Geometry: final body of the model. Coordinates: model frame, mm. A direction names the side the tool comes from. Give positions to 0.01 mm unless a question says otherwise; leave off trailing zeros. Loops run counter-clockwise (first coordinate to the right, second up) from the corner with the lowest first, then second, coordinate; pieces in that order, holes last. Notation, with made-up numbers: (-18.75, -5.75) -> (34.25, -5.75) arc R5 cw to (34.25, -1.75) -> close; hole circle Ø9 at (6.5, 17.25). An arc over 180 degrees is marked (long way). Answer in a Markdown table with one row per item. Add a question column.
1) Draft query along X for faces 1 (the flat face through (22.5, 51, -7)), 2 (the cylindrical face through (5.24, 58.166, -18.517)), 3 (the flat face through (1, 48, -18)). Return one class per face: +X half, -X half, draft (parallel to the pull), parting line (faces both ways), or undercut.
2) Section query A-A (z = -20.5). Return the cut outline in (x, y).
3) First-contact query: P1, Ø6.5, axis at x = 25.5, z = -20.5, coming from the +Y side; P2, Ø1, axis at y = 52.5, z = -14, coming from the +X side; P3, Ø1, axis at x = 9.5, z = -14.5, coming from the +Y side; P4, Ø2, axis at x = 20, y = 55.5, coming from the +Z side. Flat tips, straight axial feed; report the tip coordinate or a pass-through.
4) Line query: line 1 (X direction, y = 57.6, z = -20.5); line 2 (Y direction, x = 27, z = -18); line 3 (X direction, y = 52, z = -13.25). Output: solid intervals per line, ascending. Write a range as from..to.
5) Access query for faces 4 (the flat face through (3, 57, -21)), 5 (the flat face through (8.5, 58, -21)), 6 (the flat face through (5, 54, -27.5)), 7 (the flat face through (16, 52, -33.5)), 8 (the flat face through (5, 54, -16.5)). Directions: +Z, -Z, +X, -X, +Y, -Y. A direction counts if a zero-diameter tool reaches every point of the face in a straight line with its end or side. Return the directions, or none.
6) Section query D-D (x = 19.5). Return the cut outline in (y, z).
7) Section query C-C (x = 25.5). Return the cut outline in (y, z), plus the area to 3 significant figures.
8) Section query B-B (y = 54.25). Return the cut outline in (x, z).
```python
from build123d import *

# Parameters (mm, degrees)
BOX227_W          = 10
BOX227_H          = 10
BOX227_DEPTH      = 4
BOX217_W          = 13
BOX217_H          = 2
BOX217_DEPTH      = 1
BOX213_W          = 1
BOX213_H          = 2
BOX213_DEPTH      = 28
BOX210_W          = 2
BOX210_H          = 1
BOX210_DEPTH      = 28
BOX215_W          = 13
BOX215_H          = 2
BOX215_DEPTH      = 1
BOX212_W          = 12
BOX212_H          = 1
BOX212_DEPTH      = 2
BOX211_W          = 12
BOX211_H          = 1
BOX211_DEPTH      = 2
CYLINDER092_R     = 2
CYLINDER092_DEPTH = 5
CYLINDER093_R     = 4
CYLINDER093_DEPTH = 5
BOX073_W          = 30
BOX073_H          = 4
BOX073_DEPTH      = 30
FILLET057_R       = 6
CYLINDER088_R     = 2
CYLINDER088_DEPTH = 5
BOX221_W          = 6
BOX221_H          = 2.3
BOX221_DEPTH      = 14
FILLET055_R       = 2
BOX209_W          = 6
BOX209_H          = 7
BOX209_DEPTH      = 3
BOX222_W          = 6
BOX222_H          = 7
BOX222_DEPTH      = 3
FILLET059_R       = 1.5


with BuildPart() as cube215:
    # Box227 → Box227 (new body)
    with BuildSketch(Plane(origin=(28, 40, -16), x_dir=(1, 0, 0), z_dir=(0, 0, 1))):
        with Locations((5, 5)):
            Rectangle(BOX227_W, BOX227_H)
    extrude(amount=BOX227_DEPTH)


with BuildPart() as cube206:
    # Box217 → Box217 (new body)
    with BuildSketch(Plane(origin=(9.5, 51, -34.5), x_dir=(1, 0, 0), z_dir=(0, 0, 1))):
        with Locations((6.5, 1)):
            Rectangle(BOX217_W, BOX217_H)
    extrude(amount=BOX217_DEPTH)


with BuildPart() as cube202:
    # Box213 → Box213 (new body)
    with BuildSketch(Plane(origin=(8.5, 51, -34.5), x_dir=(1, 0, 0), z_dir=(0, 0, 1))):
        with Locations((0.5, 1)):
            Rectangle(BOX213_W, BOX213_H)
    extrude(amount=BOX213_DEPTH)


with BuildPart() as cube199:
    # Box210 → Box210 (new body)
    with BuildSketch(Plane(origin=(8.5, 50, -34.5), x_dir=(1, 0, 0), z_dir=(0, 0, 1))):
        with Locations((1, 0.5)):
            Rectangle(BOX210_W, BOX210_H)
    extrude(amount=BOX210_DEPTH)


with BuildPart() as cube204:
    # Box215 → Box215 (new body)
    with BuildSketch(Plane(origin=(9.5, 51, -7.5), x_dir=(1, 0, 0), z_dir=(0, 0, 1))):
        with Locations((6.5, 1)):
            Rectangle(BOX215_W, BOX215_H)
    extrude(amount=BOX215_DEPTH)


with BuildPart() as cube201:
    # Box212 → Box212 (new body)
    with BuildSketch(Plane(origin=(10.5, 50, -8.5), x_dir=(1, 0, 0), z_dir=(0, 0, 1))):
        with Locations((6, 0.5)):
            Rectangle(BOX212_W, BOX212_H)
    extrude(amount=BOX212_DEPTH)


with BuildPart() as fusion070:
    # Box211 → Box211 (new body)
    with BuildSketch(Plane(origin=(10.5, 50, -34.5), x_dir=(1, 0, 0), z_dir=(0, 0, 1))):
        with Locations((6, 0.5)):
            Rectangle(BOX211_W, BOX211_H)
    extrude(amount=BOX211_DEPTH)

    # Fusion070: union Cube206, Cube202, Cube199, Cube204, Cube201
    add(cube206.part)
    add(cube202.part)
    add(cube199.part)
    add(cube204.part)
    add(cube201.part)


with BuildPart() as cylinder173:
    # Cylinder092 → Cylinder092 (new body)
    with BuildSketch(Plane(origin=(25.5, 50, -20.5), x_dir=(1, 0, 0), z_dir=(0, -1, 0))):
        Circle(CYLINDER092_R)
    extrude(amount=CYLINDER092_DEPTH)


with BuildPart() as cylinder174:
    # Cylinder093 → Cylinder093 (new body)
    with BuildSketch(Plane(origin=(25.5, 47, -20.5), x_dir=(1, 0, 0), z_dir=(0, -1, 0))):
        Circle(CYLINDER093_R)
    extrude(amount=CYLINDER093_DEPTH)


with BuildPart() as cut118:
    # Box073 → Box073 (new body)
    with BuildSketch(Plane(origin=(1, 46, -36), x_dir=(1, 0, 0), z_dir=(0, 0, 1))):
        with Locations((15, 2)):
            Rectangle(BOX073_W, BOX073_H)
    extrude(amount=BOX073_DEPTH)

    # Fillet057
    fillet057_edges = [cut118.edges().sort_by_distance(p)[0] for p in [
        (1, 48, -36),
        (31, 48, -36),
    ]]
    fillet(fillet057_edges, radius=FILLET057_R)

    # Cut117: cut Cylinder174
    add(cylinder174.part, mode=Mode.SUBTRACT)

    # Cut118: cut Cylinder173
    add(cylinder173.part, mode=Mode.SUBTRACT)


with BuildPart() as cylinder169:
    # Cylinder088 → Cylinder088 (new body)
    with BuildSketch(Plane(origin=(5.5, 60, -20.5), x_dir=(1, 0, 0), z_dir=(0, -1, 0))):
        Circle(CYLINDER088_R)
    extrude(amount=CYLINDER088_DEPTH)


with BuildPart() as fillet055:
    # Box221 → Box221 (new body)
    with BuildSketch(Plane(origin=(2.5, 57, -27.5), x_dir=(1, 0, 0), z_dir=(0, 0, 1))):
        with Locations((3, 1.15)):
            Rectangle(BOX221_W, BOX221_H)
    extrude(amount=BOX221_DEPTH)

    # Cut112: cut Cylinder169
    add(cylinder169.part, mode=Mode.SUBTRACT)

    # Fillet055
    fillet055_edges = [fillet055.edges().sort_by_distance(p)[0] for p in [
        (5.5, 59.3, -13.5),
        (5.5, 59.3, -27.5),
    ]]
    fillet(fillet055_edges, radius=FILLET055_R)


with BuildPart() as cube198:
    # Box209 → Box209 (new body)
    with BuildSketch(Plane(origin=(2.5, 50, -16.5), x_dir=(1, 0, 0), z_dir=(0, 0, 1))):
        with Locations((3, 3.5)):
            Rectangle(BOX209_W, BOX209_H)
    extrude(amount=BOX209_DEPTH)


with BuildPart() as fillet059:
    # Box222 → Box222 (new body)
    with BuildSketch(Plane(origin=(2.5, 50, -27.5), x_dir=(1, 0, 0), z_dir=(0, 0, 1))):
        with Locations((3, 3.5)):
            Rectangle(BOX222_W, BOX222_H)
    extrude(amount=BOX222_DEPTH)

    # Fusion068: union Fillet055, Cube198
    add(fillet055.part)
    add(cube198.part)

    # Fusion072: union Fusion070, Cut118
    add(fusion070.part)
    add(cut118.part)

    # Cut119: cut Cube215
    add(cube215.part, mode=Mode.SUBTRACT)

    # Fillet059
    fillet059_edges = [fillet059.edges().sort_by_distance(p)[0] for p in [
        (31, 48, -16),
    ]]
    fillet(fillet059_edges, radius=FILLET059_R)


solid = fillet059.part
```
Evaluation:
| question | item | result |
|---|---|---|
| 1 | face 1 | +X half |
| 1 | face 2 | undercut |
| 1 | face 3 | -X half |
| 2 | outline | (1, 46) -> (21.5, 46) -> (21.5, 47) -> (23.5, 47) -> (23.5, 50) -> (10.5, 50) -> (10.5, 51) -> (9.5, 51) -> (9.5, 53) -> (8.5, 53) -> (8.5, 50) -> (1, 50) -> close; (2.5, 57) -> (3.5, 57) -> (3.5, 59.3) -> (2.5, 59.3) -> close; (7.5, 57) -> (8.5, 57) -> (8.5, 59.3) -> (7.5, 59.3) -> close; (27.5, 47) -> (29.5, 47) -> (29.5, 46) -> (31, 46) -> (31, 50) -> (27.5, 50) -> close |
| 3 | P1 | y = 50 |
| 3 | P2 | x = 9.5 |
| 3 | P3 | y = 53 |
| 3 | P4 | through |
| 4 | line 1 | 2.5..3.5, 7.5..8.5 |
| 4 | line 2 | 47..50 |
| 4 | line 3 | 8.5..9.5 |
| 5 | face 4 | +X, -X |
| 5 | face 5 | +Z, -Z, +X, +Y |
| 5 | face 6 | -Z, -X, +Y |
| 5 | face 7 | +X, +Y |
| 5 | face 8 | -X |
| 6 | outline | (46, -36) -> (50, -36) -> (50, -34.5) -> (53, -34.5) -> (53, -33.5) -> (51, -33.5) -> (51, -32.5) -> (50, -32.5) -> (50, -8.5) -> (51, -8.5) -> (51, -7.5) -> (53, -7.5) -> (53, -6.5) -> (50, -6.5) -> (50, -6) -> (46, -6) -> close |
| 7 | outline | (46, -35.98) -> (50, -35.98) -> (50, -22.5) -> (47, -22.5) -> (47, -24.5) -> (46, -24.5) -> close; (46, -16.5) -> (47, -16.5) -> (47, -18.5) -> (50, -18.5) -> (50, -6) -> (46, -6) -> close |
| 7 | area | 99.9 mm² |
| 8 | outline | (2.5, -27.5) -> (8.5, -27.5) -> (8.5, -24.5) -> (2.5, -24.5) -> close; (2.5, -16.5) -> (8.5, -16.5) -> (8.5, -13.5) -> (2.5, -13.5) -> close |
